from build123d import *

# Parameters (mm, degrees)
EXTRUDE_1_DEPTH = 0.5
EXTRUDE_2_DEPTH = 3
SKETCH_3_W      = 3.5
SKETCH_3_H      = 1.5
EXTRUDE_3_DEPTH = 0.2
FILLET_1_R      = 0.1


with BuildPart() as part:
    # 草图1 → 凸台-拉伸1 (new body)
    with BuildSketch(Plane.XY):
        with BuildLine():
            Line((3.4, 2.1), (-3.4, 2.1))
            ThreePointArc((-3.4, 2.1), (-5.5, 0), (-3.4, -2.1))
            Line((-3.4, -2.1), (3.4, -2.1))
            ThreePointArc((3.4, -2.1), (5.5, 0), (3.4, 2.1))
        make_face()
    extrude(amount=EXTRUDE_1_DEPTH)

    # 草图2 → 凸台-拉伸2 (add)
    with BuildSketch(Plane.XY.offset(0.5)):
        with BuildLine():
            Line((-3.4, 1.6), (3.4, 1.6))
            ThreePointArc((3.4, 1.6), (5, 0), (3.4, -1.6))
            Line((3.4, -1.6), (-3.4, -1.6))
            ThreePointArc((-3.4, -1.6), (-5, 0), (-3.4, 1.6))
        make_face()
    extrude(amount=EXTRUDE_2_DEPTH)

    # 草图3 → 凸台-拉伸3 (add)
    with BuildSketch(Plane(origin=(0, 0, 0), x_dir=(-1, 0, 0), z_dir=(0, 0, -1))):
        with Locations((-4.25, 0)):
            Rectangle(SKETCH_3_W, SKETCH_3_H)
        with Locations((4.25, 0)):
            Rectangle(SKETCH_3_W, SKETCH_3_H)
    extrude(amount=EXTRUDE_3_DEPTH)

    # 圆角1
    # the kernel refuses this fillet: 0.1 mm, written as the material it adds along each edge
    with BuildSketch(Plane(origin=(3.4, 0, 0.5), x_dir=(0, 1, 0), z_dir=(-1, 0, 0))) as fillet_1_piece_1:
        with BuildLine():
            CenterArc((1.6 + FILLET_1_R, -FILLET_1_R), FILLET_1_R, 90, 90)
            Line((1.6, -FILLET_1_R), (1.6, 0))
            Line((1.6, 0), (1.6 + FILLET_1_R, 0))
        make_face()
    revolve(axis=Axis((3.4, 0, 0.5), (0, 0, -1)), revolution_arc=180)
    with BuildSketch(Plane(origin=(-3.4, 1.6, 0.5), x_dir=(0, 1, 0), z_dir=(1, 0, 0)), Plane(origin=(3.4, -1.6, 0.5), x_dir=(0, -1, 0), z_dir=(-1, 0, 0))) as fillet_1_piece_2:
        with BuildLine():
            CenterArc((FILLET_1_R, FILLET_1_R), FILLET_1_R, 180, 90)
            Line((0, FILLET_1_R), (0, 0))
            Line((0, 0), (FILLET_1_R, 0))
        make_face()
    extrude(amount=6.8)
    with BuildSketch(Plane(origin=(-3.4, 0, 0.5), x_dir=(0, -1, 0), z_dir=(1, 0, 0))) as fillet_1_piece_3:
        with BuildLine():
            CenterArc((1.6 + FILLET_1_R, -FILLET_1_R), FILLET_1_R, 90, 90)
            Line((1.6, -FILLET_1_R), (1.6, 0))
            Line((1.6, 0), (1.6 + FILLET_1_R, 0))
        make_face()
    revolve(axis=Axis((-3.4, 0, 0.5), (0, 0, -1)), revolution_arc=180)
    # the kernel refuses this fillet: 0.1 mm, written as the material it takes off along each edge
    with BuildSketch(Plane(origin=(-3.4, 0, 0.5), x_dir=(0, 1, 0), z_dir=(1, 0, 0))) as fillet_1_2_piece_1:
        with BuildLine():
            CenterArc((2.1 - FILLET_1_R, -FILLET_1_R), FILLET_1_R, 0, 90)
            Line((2.1 - FILLET_1_R, 0), (2.1, 0))
            Line((2.1, 0), (2.1, -FILLET_1_R))
        make_face()
    revolve(axis=Axis((-3.4, 0, 0.5), (0, 0, 1)), revolution_arc=180, mode=Mode.SUBTRACT)
    with BuildSketch(Plane(origin=(-3.4, -2.1, 0.5), x_dir=(0, 1, 0), z_dir=(1, 0, 0)), Plane(origin=(-3.4, 1.6, 3.5), x_dir=(0, 0, -1), z_dir=(1, 0, 0)), Plane(origin=(3.4, -1.6, 3.5), x_dir=(0, 0, -1), z_dir=(-1, 0, 0))) as fillet_1_2_piece_2:
        with BuildLine():
            CenterArc((FILLET_1_R, -FILLET_1_R), FILLET_1_R, 90, 90)
            Line((0, -FILLET_1_R), (0, 0))
            Line((0, 0), (FILLET_1_R, 0))
        make_face()
    extrude(amount=6.8, mode=Mode.SUBTRACT)
    with BuildSketch(Plane(origin=(3.4, 0, 3.5), x_dir=(0, 1, 0), z_dir=(-1, 0, 0))) as fillet_1_2_piece_3:
        with BuildLine():
            CenterArc((1.6 - FILLET_1_R, FILLET_1_R), FILLET_1_R, 270, 90)
            Line((1.6 - FILLET_1_R, 0), (1.6, 0))
            Line((1.6, 0), (1.6, FILLET_1_R))
        make_face()
    revolve(axis=Axis((3.4, 0, 3.5), (0, 0, -1)), revolution_arc=180, mode=Mode.SUBTRACT)
    with BuildSketch(Plane(origin=(-3.4, 0, 3.5), x_dir=(0, -1, 0), z_dir=(1, 0, 0))) as fillet_1_2_piece_4:
        with BuildLine():
            CenterArc((1.6 - FILLET_1_R, FILLET_1_R), FILLET_1_R, 270, 90)
            Line((1.6 - FILLET_1_R, 0), (1.6, 0))
            Line((1.6, 0), (1.6, FILLET_1_R))
        make_face()
    revolve(axis=Axis((-3.4, 0, 3.5), (0, 0, -1)), revolution_arc=180, mode=Mode.SUBTRACT)
    with BuildSketch(Plane(origin=(-3.4, 0, 0), x_dir=(-0.9698622672900031, -0.2436538168941636, 0), z_dir=(-0.2436538168941636, 0.9698622672900031, 0))) as fillet_1_2_piece_5_section:
        with BuildLine():
            CenterArc((2.1 - FILLET_1_R, FILLET_1_R), FILLET_1_R, 270, 90)
            Line((2.1 - FILLET_1_R, 0), (2.1, 0))
            Line((2.1, 0), (2.1, FILLET_1_R))
        make_face()
    fillet_1_2_piece_5 = revolve(axis=Axis((-3.4, 0, 0), (0, 0, 1)), revolution_arc=75.897707553, mode=Mode.PRIVATE)
    fillet_1_2_piece_5 = split(fillet_1_2_piece_5, bisect_by=Plane(origin=(-4.574684064, -0.75, 0.028052066), z_dir=(0, -1, 0)), keep=Keep.TOP, mode=Mode.PRIVATE)
    add(fillet_1_2_piece_5, mode=Mode.SUBTRACT)
    with BuildSketch(Plane(origin=(3.4, 0, 0.5), x_dir=(0, -1, 0), z_dir=(-1, 0, 0))) as fillet_1_2_piece_6:
        with BuildLine():
            CenterArc((2.1 - FILLET_1_R, -FILLET_1_R), FILLET_1_R, 0, 90)
            Line((2.1 - FILLET_1_R, 0), (2.1, 0))
            Line((2.1, 0), (2.1, -FILLET_1_R))
        make_face()
    revolve(axis=Axis((3.4, 0, 0.5), (0, 0, 1)), revolution_arc=180, mode=Mode.SUBTRACT)
    with BuildSketch(Plane(origin=(-3.4, -2.1, 0), x_dir=(0, 1, 0), z_dir=(1, 0, 0)), Plane(origin=(3.4, 2.1, 0.5), x_dir=(0, 0, -1), z_dir=(-1, 0, 0))) as fillet_1_2_piece_7:
        with BuildLine():
            CenterArc((FILLET_1_R, FILLET_1_R), FILLET_1_R, 180, 90)
            Line((0, FILLET_1_R), (0, 0))
            Line((0, 0), (FILLET_1_R, 0))
        make_face()
    extrude(amount=6.8, mode=Mode.SUBTRACT)
    with BuildSketch(Plane(origin=(3.4, 0, 0), x_dir=(0, -1, 0), z_dir=(-1, 0, 0))) as fillet_1_2_piece_8_section:
        with BuildLine():
            CenterArc((2.1 - FILLET_1_R, FILLET_1_R), FILLET_1_R, 270, 90)
            Line((2.1 - FILLET_1_R, 0), (2.1, 0))
            Line((2.1, 0), (2.1, FILLET_1_R))
        make_face()
    fillet_1_2_piece_8 = revolve(axis=Axis((3.4, 0, 0), (0, 0, 1)), revolution_arc=75.897707553, mode=Mode.PRIVATE)
    fillet_1_2_piece_8 = split(fillet_1_2_piece_8, bisect_by=Plane(origin=(4.574684074, -0.75, 0.028052047), z_dir=(0, -1, 0)), keep=Keep.TOP, mode=Mode.PRIVATE)
    add(fillet_1_2_piece_8, mode=Mode.SUBTRACT)


solid = part.part
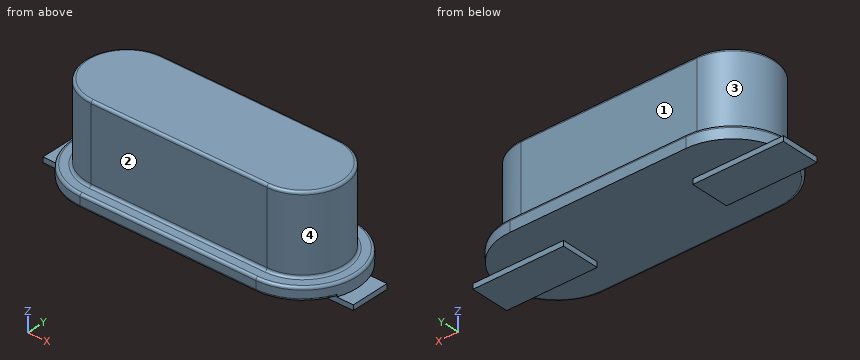
The model under review builds one solid part; all positions refer to its coordinate system, in mm. Face numbers are marked on the shaded views. A direction names the side the tool comes from. Give positions to 0.01 mm unless a question says otherwise; leave off trailing zeros. Loops run counter-clockwise (first coordinate to the right, second up) from the corner with the lowest first, then second, coordinate; pieces in that order, holes last. Notation, with made-up numbers: (72.5, 63) -> (122.5, 63) arc R11 cw to (122.5, 81) -> close; hole circle Ø9 at (-17, 64). An arc over 180 degrees is marked (long way). Put each result on its own line as item: value. Start each with the question number.
1. Clearance check with flat-ended pins moving along their axes: P1, Ø1.5, axis at y = -1.5, z = 1.5, coming from the -X side; P2, Ø1.2, axis at x = 1, y = 0, coming from the -Z side; P3, Ø1.5, axis at y = -1, z = 1.5, coming from the -X side. State where each tip first meets the part, or that it passes through.
2. We need section A-A on x = -1.25. State the section outline as (y, z) points.
3. We need section C-C on z = 1.6. State the section outline as (x, y) points.
4. Wall thickness on probe 1 along Y at (x, z) = (0, 2.65); probe 2 along Z at (x, y) = (-0.75, 0); probe 3 along X at (y, z) = (0, 3.15): over which ranges is each line inside the solid? List them lowest first.
5. We need section B-B on y = 0. State the section outline as (x, z) points.
6. For the marked faces 1, 2, 3 and 4, list the 3-axis set-ups (+Z, -Z, +X, -X, +Y, -Y) from which the entire face can be reached by the end or side of a thin tool; tool diameter is ignored.
Determined:
1. P1: x = -4.81
1. P2: z = 0
1. P3: x = -4.98
2. outline: (-2.1, 0.1) arc R0.1 ccw to (-2, 0) -> (2.1, 0) -> (2.1, 0.4) arc R0.1 ccw to (2, 0.5) -> (1.7, 0.5) arc R0.1 cw to (1.6, 0.6) -> (1.6, 3.4) arc R0.1 ccw to (1.5, 3.5) -> (-1.5, 3.5) arc R0.1 ccw to (-1.6, 3.4) -> (-1.6, 0.6) arc R0.1 cw to (-1.7, 0.5) -> (-2, 0.5) arc R0.1 ccw to (-2.1, 0.4) -> close
3. outline: (-3.4, -1.6) -> (3.4, -1.6) arc R1.6 ccw to (3.4, 1.6) -> (-3.4, 1.6) arc R1.6 ccw to start
4. probe 1: -1.6 to 1.6
4. probe 2: 0 to 3.5
4. probe 3: -5 to 5
5. outline: (-6, -0.2) -> (-2.5, -0.2) -> (-2.5, 0) -> (2.5, 0) -> (2.5, -0.2) -> (6, -0.2) -> (6, 0) -> (5.5, 0) -> (5.5, 0.4) arc R0.1 ccw to (5.4, 0.5) -> (5.1, 0.5) arc R0.1 cw to (5, 0.6) -> (5, 3.4) arc R0.1 ccw to (4.9, 3.5) -> (-4.9, 3.5) arc R0.1 ccw to (-5, 3.4) -> (-5, 0.6) arc R0.1 cw to (-5.1, 0.5) -> (-5.4, 0.5) arc R0.1 ccw to (-5.5, 0.4) -> (-5.5, 0) -> (-6, 0) -> close
6. face 1: +Z, +X, -X, +Y
6. face 2: +Z, +X, -X, -Y
6. face 3: +Z, -X
6. face 4: +Z, +X
